from build123d import *

# Parameters (mm, degrees)
SKETCH_1_W          = 47
SKETCH_1_H          = 3
EXTRUDE_1_DEPTH     = 25
SKETCH_2_R          = 1.75
SKETCH_2_R_2        = 28.55
CUT_EXTRUDE_1_DEPTH = 4


with BuildPart() as part:
    # 草圖1 → 填料-伸長1 (new body, symmetric)
    with BuildSketch(Plane(origin=(0, 0, 0), x_dir=(0, 0, -1), z_dir=(1, 0, 0))):
        Polygon((0, 50), (0, 0), (3, 0), (3, 3), (3, 50), align=None)
        with Locations((26.5, 1.5)):
            Rectangle(SKETCH_1_W, SKETCH_1_H)
    extrude(amount=EXTRUDE_1_DEPTH, both=True)

    # 草圖2 → 除料-伸長1 (cut, through all)
    with BuildSketch(Plane(origin=(0, 0, -3), x_dir=(-1, 0, 0), z_dir=(0, 0, -1))):
        with Locations((17, 10.172548614)):
            Circle(SKETCH_2_R)
        with Locations((-17, 10.172548614)):
            Circle(SKETCH_2_R)
        with Locations((-34, 39.617412342)):
            Circle(SKETCH_2_R)
        with Locations((-17, 69.062276071)):
            Circle(SKETCH_2_R)
        with Locations((17, 69.062276071)):
            Circle(SKETCH_2_R)
        with Locations((34, 39.617412342)):
            Circle(SKETCH_2_R)
        with Locations((0, 39.617412342)):
            Circle(SKETCH_2_R_2)
    extrude(amount=-CUT_EXTRUDE_1_DEPTH, mode=Mode.SUBTRACT)


solid = part.part
CAD build for the part. Positions are in the model's coordinates, mm. A direction names the side the tool comes from. Round coordinates to 2 decimals unless told otherwise and drop trailing zeros. Order: outer loops, then holes, each group sorted by start corner. A loop starts at its lowest first (then second) coordinate and runs counter-clockwise, first axis right, second up. Notation, with made-up numbers: (54.25, 18.5) - (107.25, 18.5) arc R22 ccw to (107.25, 26.5) - close; hole circle Ø1 at (31.5, 52). An arc over 180 degrees is marked (long way). Return JSON: item names as keys, results as strings.
(1) Tool access for faces 1 (the face through (0, 1, -50)), 2 (the face through (0, 9, -3)): list every direction of +Z, -Z, +X, -X, +Y, -Y with a clear straight run to the whole face (end or side of a thin tool).
Answer key:
{"face 1": "-Z, +X, -X, +Y, -Y", "face 2": "-Z, +X, -X, +Y"}
(2) Cut at C-C (z = -6). Give the cut face in (x, y), then the cut area to 3 significant figures.
Answer key:
{"outline": "(-25, 0) - (25, 0) - (25, 3) - (-25, 3) - close", "area": "150 mm^2"}
(3) Cut at B-B (x = 17). Give the cut face in (y, z).
Answer key:
{"outline": "(0, -50) - (3, -50) - (3, -3) - (8.42, -3) - (8.42, 0) - (0, 0) - close; (11.92, -3) - (16.68, -3) - (16.68, 0) - (11.92, 0) - close"}
(4) Cut at A-A (y = 19.25). Give the cut face in (x, z).
Answer key:
{"outline": "(-25, -3) - (-20.01, -3) - (-20.01, 0) - (-25, 0) - close; (20.01, -3) - (25, -3) - (25, 0) - (20.01, 0) - close"}
(5) Cut at D-D (y = 6.25). Give the cut face in (x, z), then the cut area to 3 significant figures.
Answer key:
{"outline": "(-25, -3) - (25, -3) - (25, 0) - (-25, 0) - close", "area": "150 mm^2"}
(6) Wall check: probe 1 along X at (y, z) = (10.5, -2.5); probe 2 along Y at (x, z) = (-17, -1.6); probe 3 along Y at (x, z) = (-12, -19). Give the ranges that are in metal, low to high. Write a range as from..to.
Answer key:
{"probe 1": "x = -25..-18.72, -15.28..15.28, 18.72..25", "probe 2": "y = 0..8.42, 11.92..16.68", "probe 3": "y = 0..3"}
(7) Pull direction X, two halves, no side cores. Call faces 3 (the face through (-25, 2, -16)), 4 (the face through (25, 2, -16)), 5 (the face through (18.29, 11.355, -1.521)): +X half, -X half, draft (parallel to the pull), parting line (faces both ways), or undercut.
Answer key:
{"face 3": "-X half", "face 4": "+X half", "face 5": "undercut"}
(8) Pin check, flat tips, straight feed: pin 1 Ø2 at (x, y) = (8.5, 7.5) entering from -Z; pin 2 Ø2 at (x, z) = (8, -38.5) entering from +Y. Stop position of each tip, or through.
Answer key:
{"pin 1": "stops at z = -3", "pin 2": "stops at y = 3"}
